from build123d import *

# Parameters (mm, degrees)
BOSS_EXTRUDE2_DEPTH = 5
SKETCH3_R           = 3.25
CUT_EXTRUDE1_DEPTH  = 11
SKETCH4_W           = 13
SKETCH4_H           = 7
BOSS_EXTRUDE3_DEPTH = 2.5
SKETCH5_R           = 2.5
CUT_EXTRUDE2_DEPTH  = 8.5
SKETCH6_W           = 7
SKETCH6_H           = 10
SKETCH6_R           = 3.25
BOSS_EXTRUDE4_DEPTH = 30


with BuildPart() as part:
    # Sketch2 → Boss-Extrude2 (new body, symmetric)
    with BuildSketch(Plane.XY):
        Polygon((0, 0), (-7, 0), (-17, 10), (-10, 10), align=None)
    extrude(amount=BOSS_EXTRUDE2_DEPTH, both=True)

    # Sketch3 → Cut-Extrude1 (cut, through all)
    with BuildSketch(Plane.XZ):
        with Locations((-3.5, 0)):
            Circle(SKETCH3_R)
    extrude(amount=-CUT_EXTRUDE1_DEPTH, mode=Mode.SUBTRACT)

    # Sketch4 → Boss-Extrude3 (add, symmetric)
    with BuildSketch(Plane.XY):
        with Locations((-16.5, 6.5)):
            Rectangle(SKETCH4_W, SKETCH4_H)
    extrude(amount=BOSS_EXTRUDE3_DEPTH, both=True)

    # Sketch5 → Cut-Extrude2 (cut, through all)
    with BuildSketch(Plane.XY.offset(2.5)):
        with Locations((-20, 6.5)):
            Circle(SKETCH5_R)
    extrude(amount=-CUT_EXTRUDE2_DEPTH, mode=Mode.SUBTRACT)

    # Sketch6 → Boss-Extrude4 (add)
    with BuildSketch(Plane.XZ):
        with Locations((-3.5, 0)):
            Rectangle(SKETCH6_W, SKETCH6_H)
        with Locations((-3.5, 0)):
            Circle(SKETCH6_R, mode=Mode.SUBTRACT)
    extrude(amount=BOSS_EXTRUDE4_DEPTH)


solid = part.part
Here's how the part is built. I have some questions about the finished solid (model axes, mm). A direction names the side the tool comes from. Round coordinates to 2 decimals unless told otherwise and drop trailing zeros. Write each loop counter-clockwise with the first axis right and the second up, starting at its lowest first coordinate (ties: lowest second). Pieces come first, ordered by that corner, then holes.
1. I need wall thicknesses on L1, parallel to Z at x = -3.5, y = -16.25; L2, parallel to Y at x = -20, z = 0.2; L3, parallel to X at y = -7, z = -1.25. Which ranges of each line are inside material? Lowest first, please.
2. Suppose I cut it at C-C (y = -26). List the corners of the cut face in (x, z) for me.
3. For faces 4 (the flat face through (-17, 6, 2.5)), 5 (the flat face through (-5, -10, 5)), 6 (the flat face through (-7, -15, 0)), which set-ups out of +Z, -Z, +X, -X, +Y, -Y let a thin tool reach every point of the face, with its end or its side?
4. Suppose I cut it at D-D (x = -16.5). List the corners of the cut face in (y, z) for me, and give its area (3 significant figures).
5. If we mould it in two halves opening along Y, with no side actions, what happens to faces 1 (the cylindrical face through (-22.5, 6.6, 0)), 2 (the flat face through (-17, 3, 0)), 3 (the flat face through (-17, 6, -2.5))? For each: released by +Y, released by -Y, zero draft, split by the parting line, or undercut.
6. Suppose I cut it at B-B (z = 0). List the corners of the cut face in (x, y) for me, and give its area (3 significant figures).
7. Suppose I cut it at A-A (x = -3.5). List the corners of the cut face in (y, z) for me, and give its area (3 significant figures).
8. Will these pins go through, and if not, where does the flat tip stop? pin 1 Ø5 at (x, z) = (-3.5, 0) entering from +Y; pin 2 Ø6.5 at (x, y) = (-20, 6.5) entering from -Z; pin 3 Ø1 at (y, z) = (0, -3.5) entering from -X; pin 4 Ø5 at (y, z) = (-15.5, -1) entering from -X.
Answer sheet:
1. L1: z = -5 to -3.25, 3.25 to 5
1. L2: y = 3 to 4, 9 to 10
1. L3: x = -7 to -6.5, -0.5 to 0
2. outline: (-7, -5) - (0, -5) - (0, 5) - (-7, 5) - close; hole circle Ø6.5 at (-3.5, 0)
3. face 4: +Z, -X, -Y
3. face 5: +Z, +X, -X, +Y, -Y
3. face 6: +Z, -Z, -X, -Y
4. outline: (3, -2.5) - (9.5, -2.5) - (9.5, -5) - (10, -5) - (10, 5) - (9.5, 5) - (9.5, 2.5) - (3, 2.5) - close
4. area: 37.5 mm2
5. face 1: undercut
5. face 2: released by -Y
5. face 3: zero draft
6. outline: (-23, 3) - (-10, 3) - (-7, 0) - (-7, -30) - (-6.75, -30) - (-6.75, 6.75) - (-10, 10) - (-23, 10) - close; (-0.25, -30) - (0, -30) - (0, 0) - (-0.25, 0.25) - close; hole circle Ø5 at (-20, 6.5)
6. area: 109 mm2
7. outline: (-30, -5) - (3.5, -5) - (3.5, -3.25) - (-30, -3.25) - close; (-30, 3.25) - (3.5, 3.25) - (3.5, 5) - (-30, 5) - close
7. area: 117 mm2
8. pin 1: passes through
8. pin 2: stops at z = -2.5
8. pin 3: stops at x = -7.5
8. pin 4: stops at x = -7
